Could you check a few things on this model? Use its own coordinates, in mm. Face numbers are marked on the shaded views. A direction names the side the tool comes from. Give positions to 0.01 mm unless a question says otherwise; leave off trailing zeros. Order: outer loops, then holes, each group sorted by start corner. A loop starts at its lowest first (then second) coordinate and runs counter-clockwise, first axis right, second up. Notation, with made-up numbers: (-26, -30) - (3, -30) arc R25 ccw to (3, -15) - close; hole circle Ø6 at (71.5, -30.75). An arc over 180 degrees is marked (long way). Put each result on its own line as item: value.
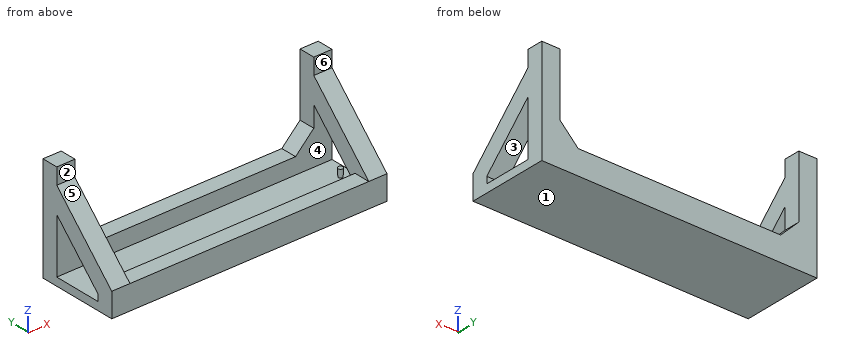
from build123d import *

# Parameters (mm, degrees)
F0_W      = 200
F0_H      = 20
F1_DEPTH  = 340
F2_W      = 40
F2_H      = 40
F3_DEPTH  = 340
F4_W      = 45
F4_H      = 40
F5_DEPTH  = 200
F7_DEPTH  = 45
F9_DEPTH  = 40
F10_R     = 5
F11_DEPTH = 20
F11_TAPER = -3


# Not quite as in the source:
# - a pattern or mirror of a feature is missing from the dataset's text; its kind, count and spacing are read off the source's solid


with BuildPart() as f1:
    # F0 (on Right) → F1 (new body, symmetric)
    with BuildSketch(Plane.YZ):
        Rectangle(F0_W, F0_H)
    extrude(amount=F1_DEPTH, both=True)

    # F2 (on Right) → F3 (join, symmetric)
    with BuildSketch(Plane.YZ):
        with Locations((80, 30)):
            Rectangle(F2_W, F2_H)
        with Locations((-80, 30)):
            Rectangle(F2_W, F2_H)
    extrude(amount=F3_DEPTH, both=True)

    # F4 (on face) → F5 (join)
    with BuildSketch(Plane.XY.offset(50)):
        with Locations((-317.5, 80)):
            Rectangle(F4_W, F4_H)
        with Locations((317.5, 80)):
            Rectangle(F4_W, F4_H)
    extrude(amount=F5_DEPTH)

    # F6 (on face) → F7 (join)
    with BuildSketch(Plane.YZ.offset(340)):
        Polygon((60, 210), (-100, 50), (-60, 50), (-60, 26.3603896932), (60, 146.3603896932), align=None)
    f7 = extrude(amount=-F7_DEPTH)

    # F7_copies: F7 across plane
    add(f7.mirror(Plane(origin=(0, 0, 0), x_dir=(0, 0, -1), z_dir=(-1, 0, 0))))

    # F8 (on face) → F9 (join)
    with BuildSketch(Plane(origin=(0, 100, 0), x_dir=(-1, 0, 0), z_dir=(0, 1, 0))):
        Polygon((-250, 50), (-295, 95), (-295, 50), align=None)
        Polygon((295, 50), (295, 95), (250, 50), align=None)
    extrude(amount=-F9_DEPTH)

    # F10 (on face) → F11 (join)
    with BuildSketch(Plane.XY.offset(10)):
        with Locations((310, 0)):
            Circle(F10_R)
    extrude(amount=F11_DEPTH, taper=F11_TAPER)


solid = f1.part
1) Suppose I cut it at A-A, the plane z = 230. List the corners of the cut face in (x, y) for me, and give its area (3 significant figures).
Filled in:
outline: (-340, 60) - (-295, 60) - (-295, 100) - (-340, 100) - close; (295, 60) - (340, 60) - (340, 100) - (295, 100) - close
area: 3,600 mm^2
2) We'd pull the mould along Z, two halves only. Please class the marked faces 3, 4, 5 and 6: pulls with the +Z half, pulls with the -Z half, needs draft (parallel to the pull), parting line crosses it, or undercut.
Filled in:
face 3: undercut
face 4: undercut
face 5: pulls with the +Z half
face 6: needs draft
3) Which directions (+Z, -Z, +X, -X, +Y, -Y) give clear straight access to the entire face, cutting with the end or side of a thin tool? Please do the marked faces 1 and 2.
Filled in:
face 1: -Z, +X, -X, +Y, -Y
face 2: +Z, +X, -X, -Y
4) If I drill on line 1 (X direction, y = 25, z = 164.5); line 2 (Y direction, x = -39.5, z = 38); line 3 (Y direction, x = 308.5, z = 26.5), over which ranges is the centre line in solid material (lowest first)? Write a range as [from, to].
Filled in:
line 1: x = [-340, -295], [295, 340]
line 2: y = [-100, -60], [60, 100]
line 3: y = [-100, -59.86], [-5.67, 5.67], [60, 100]
5) Suppose I cut it at B-B, the plane x = -73. List the corners of the cut face in (y, z) for me, and give its area (3 significant figures).
Filled in:
outline: (-100, -10) - (100, -10) - (100, 50) - (60, 50) - (60, 10) - (-60, 10) - (-60, 50) - (-100, 50) - close
area: 7,200 mm^2
6) Suppose I cut it at C-C, the plane y = 32. List the corners of the cut face in (x, z) for me, and give its area (3 significant figures).
Filled in:
outline: (-340, -10) - (340, -10) - (340, 10) - (-340, 10) - close; (-340, 118.36) - (-295, 118.36) - (-295, 182) - (-340, 182) - close; (295, 118.36) - (340, 118.36) - (340, 182) - (295, 182) - close
area: 19,300 mm^2
7) Suppose I cut it at D-D, the plane z = 78. List the corners of the cut face in (x, y) for me, and give its area (3 significant figures).
Filled in:
outline: (-340, -72) - (-295, -72) - (-295, -8.36) - (-340, -8.36) - close; (-340, 60) - (-278, 60) - (-278, 100) - (-340, 100) - close; (278, 60) - (340, 60) - (340, 100) - (278, 100) - close; (295, -72) - (340, -72) - (340, -8.36) - (295, -8.36) - close
area: 10,700 mm^2
8) I'm going to push flat-ended pins straight in: pin 1 (12 mm diameter, centred on x = -29.5, y = 88, fed in from +Z); pin 2 (12 mm diameter, centred on x = -128.5, y = -0.5, fed in from +Z); pin 3 (13.5 mm diameter, centred on x = 308.5, y = 1.5, fed in from +Z). Where does each tip first touch, or does it pass through?
Filled in:
pin 1: stops at z = 50
pin 2: stops at z = 10
pin 3: stops at z = 158.25
